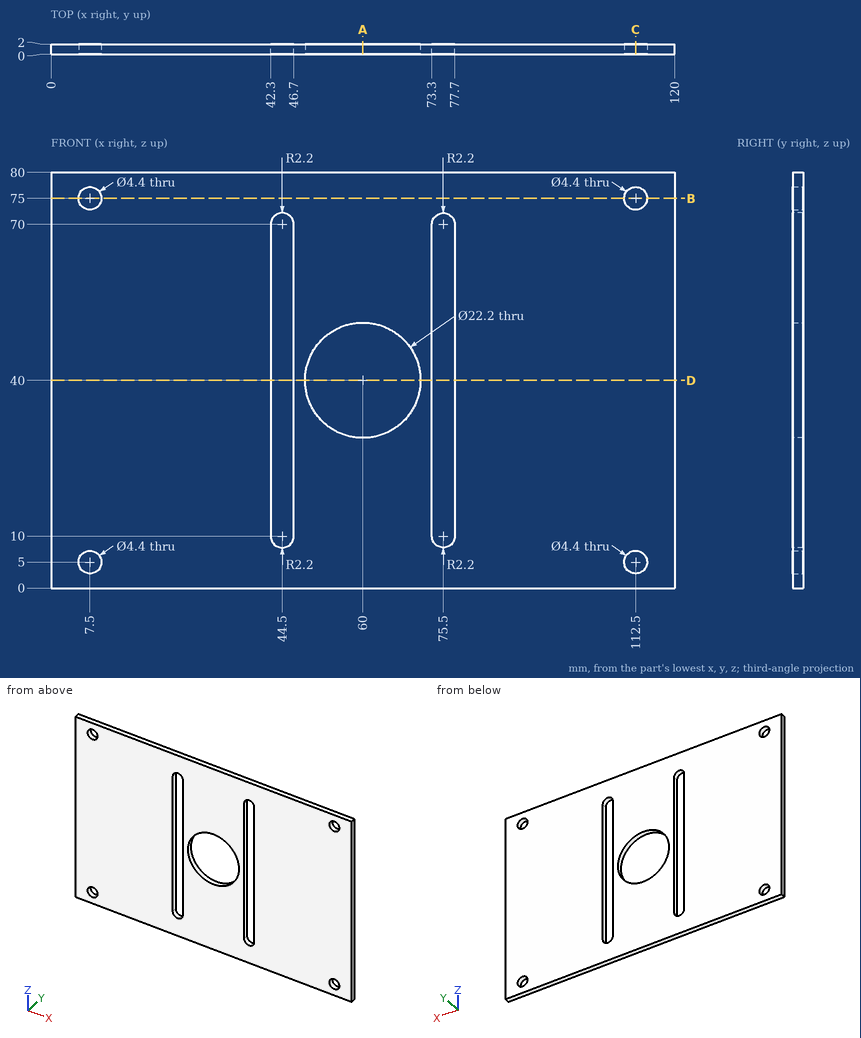
Answer from the drawing. Dimensions are ordinates in mm from the lowest x, y and z of the part. Round coordinates to 2 decimals unless told otherwise and drop trailing zeros. Write each loop counter-clockwise with the first axis right and the second up, starting at its lowest first coordinate (ties: lowest second). Pieces come first, ordered by that corner, then holes. Notation, with made-up numbers: (14, -35.75) -> (61, -35.75) arc R22 ccw to (61, -14.75) -> close; hole circle Ø9 at (3.25, -15.75). An arc over 180 degrees is marked (long way). Write each question's results on one line, items separated by ' | '.
1) The part is cut by section A-A (x = 60). Write down the section's boundary in (y, z).
Findings:
outline: (0, 0) -> (2, 0) -> (2, 28.9) -> (0, 28.9) -> close; (0, 51.1) -> (2, 51.1) -> (2, 80) -> (0, 80) -> close
2) The part is cut by section C-C (x = 112.5). Write down the section's boundary in (y, z).
Findings:
outline: (0, 0) -> (2, 0) -> (2, 2.8) -> (0, 2.8) -> close; (0, 7.2) -> (2, 7.2) -> (2, 72.8) -> (0, 72.8) -> close; (0, 77.2) -> (2, 77.2) -> (2, 80) -> (0, 80) -> close
3) The part is cut by section B-B (z = 75). Write down the section's boundary in (x, y), and give its area (3 significant figures).
Findings:
outline: (0, 0) -> (5.3, 0) -> (5.3, 2) -> (0, 2) -> close; (9.7, 0) -> (110.3, 0) -> (110.3, 2) -> (9.7, 2) -> close; (114.7, 0) -> (120, 0) -> (120, 2) -> (114.7, 2) -> close | area: 222 mm²
4) Consider line 1 along X through (y, z) = (0.8, 24.5); line 2 along Z through (x, y) = (112.5, 1.2); line 3 along X through (y, z) = (1.15, 40). Determine where each line is inside the solid, lowest interval first. Write a range as [from, to].
Findings:
line 1: x = [0, 42.3], [46.7, 73.3], [77.7, 120] | line 2: z = [0, 2.8], [7.2, 72.8], [77.2, 80] | line 3: x = [0, 42.3], [46.7, 48.9], [71.1, 73.3], [77.7, 120]
5) The part is cut by section D-D (z = 40). Write down the section's boundary in (x, y), and give its area (3 significant figures).
Findings:
outline: (0, 0) -> (42.3, 0) -> (42.3, 2) -> (0, 2) -> close; (46.7, 0) -> (48.9, 0) -> (48.9, 2) -> (46.7, 2) -> close; (71.1, 0) -> (73.3, 0) -> (73.3, 2) -> (71.1, 2) -> close; (77.7, 0) -> (120, 0) -> (120, 2) -> (77.7, 2) -> close | area: 178 mm²
